```python
from build123d import *

# Parameters (mm, degrees)
F0_W     = 82.55
F0_H     = 50.8
F0_R     = 5.5
F1_DEPTH = 19.05
F3_D     = 7.112
F4_R     = 5.08


with BuildPart() as f1:
    # F0 (on Right) → F1 (new body)
    with BuildSketch(Plane.YZ):
        Rectangle(F0_W, F0_H)
        Circle(F0_R, mode=Mode.SUBTRACT)
    extrude(amount=F1_DEPTH)

    # F3 (through all)
    with Locations(Plane.YZ.offset(19.05)):
        with Locations((-31.75, 12.7), (31.75, 12.7), (31.75, -12.7), (-31.75, -12.7)):
            Hole(F3_D / 2)

    # F4
    f4_edges = [f1.edges().sort_by_distance(p)[0] for p in [
        (9.525, -41.275, 25.4),
        (9.525, -41.275, -25.4),
        (9.525, 41.275, -25.4),
        (9.525, 41.275, 25.4),
    ]]
    fillet(f4_edges, radius=F4_R)


solid = f1.part
```
Here's how the part is built. I have some questions about the finished solid (model axes, mm). Coordinates: 2 decimals unless noted, no trailing zeros. Order: outer loops, then holes, each group sorted by start corner. A loop starts at its lowest first (then second) coordinate and runs counter-clockwise, first axis right, second up. Notation, with made-up numbers: (88.25, -11.5) - (146.25, -11.5) arc R19 ccw to (146.25, -2.5) - close; hole circle Ø11 at (-14.5, 50.5). An arc over 180 degrees is marked (long way). One line per question, with ' | ' between items.
(1) Suppose I cut it at A-A on y = 0. List the corners of the cut face in (x, z) for me, and give its area (3 significant figures).
Report:
outline: (0, -25.4) - (19.05, -25.4) - (19.05, -5.5) - (0, -5.5) - close; (0, 5.5) - (19.05, 5.5) - (19.05, 25.4) - (0, 25.4) - close | area: 758 mm2
(2) If I drill on L1, parallel to Z at x = 8.5, y = 31.75; L2, parallel to Y at x = 11.5, z = -15.5 (3 decimals); L3, parallel to Z at x = 7, y = 0, over which ranges is the centre line in solid material (lowest first)?
Report:
L1: z = -25.4 to -16.26, -9.14 to 9.14, 16.26 to 25.4 | L2: y = -41.275 to -33.942, -29.558 to 29.558, 33.942 to 41.275 | L3: z = -25.4 to -5.5, 5.5 to 25.4
(3) Suppose I cut it at C-C on z = -12.7. List the corners of the cut face in (x, y) for me (3 decimals), and give its area (3 significant figures).
Report:
outline: (0, -41.275) - (19.05, -41.275) - (19.05, -35.306) - (0, -35.306) - close; (0, -28.194) - (19.05, -28.194) - (19.05, 28.194) - (0, 28.194) - close; (0, 35.306) - (19.05, 35.306) - (19.05, 41.275) - (0, 41.275) - close | area: 1,300 mm2
(4) Suppose I cut it at D-D on x = 13. List the corners of the cut face in (y, z) for me (3 decimals), and give its area (3 significant figures).
Report:
outline: (-41.275, -20.32) arc R5.08 ccw to (-36.195, -25.4) - (36.195, -25.4) arc R5.08 ccw to (41.275, -20.32) - (41.275, 20.32) arc R5.08 ccw to (36.195, 25.4) - (-36.195, 25.4) arc R5.08 ccw to (-41.275, 20.32) - close; hole circle Ø7.112 at (-31.75, -12.7); hole circle Ø7.112 at (-31.75, 12.7); hole circle Ø11 at (0, 0); hole circle Ø7.112 at (31.75, -12.7); hole circle Ø7.112 at (31.75, 12.7) | area: 3,920 mm2
(5) Suppose I cut it at B-B on z = 0. List the corners of the cut face in (x, y) for me (3 decimals).
Report:
outline: (0, -41.275) - (19.05, -41.275) - (19.05, -5.5) - (0, -5.5) - close; (0, 5.5) - (19.05, 5.5) - (19.05, 41.275) - (0, 41.275) - close
(6) If we mould it in two halves opening along Z, with no side actions, what happens to faces 1 (the flat face through (9, -1, 25.4)), 2 (the flat face through (9, 41.275, 0)), 3 (the cylindrical face through (9.392, 34.371, 15.103)), 4 (the cylindrical face through (9.66, 39.75, -23.95))? For each: pulls with the +Z half, pulls with the -Z half, needs draft (parallel to the pull), parting line crosses it, or undercut.
Report:
face 1: pulls with the +Z half | face 2: needs draft | face 3: undercut | face 4: pulls with the -Z half
(7) Will this pin go through, and if not, where does the flat tip stop? pin 1 (5 mm diameter, centred on y = 25, z = -17.5, fed in from -X).
Report:
pin 1: stops at x = 0
